Drawing for the job (mm, zero at the part's lowest x, y, z). A direction names the side the tool comes from. Round coordinates to 2 decimals unless told otherwise and drop trailing zeros. Write each loop counter-clockwise with the first axis right and the second up, starting at its lowest first coordinate (ties: lowest second). Pieces come first, ordered by that corner, then holes. Notation, with made-up numbers: M 45,75.25 L 53,75.25 A8 ccw 53,85.25 Z; hole C -26,83 d8. An arc over 180 degrees is marked long. Use a Markdown table: item, result. Add a question column.
1) Which spindle directions (+Z, -Z, +X, -X, +Y, -Y) get a long thin tool onto all of the face, cutting with end or side? Do the marked faces 1 and 2. Say none if no direction does.
2) Wall check: probe 1 along Y at (x, z) = (22.5, 4); probe 2 along X at (y, z) = (9, 77.5); probe 3 along Y at (x, z) = (7, 47). Give the ranges that are in metal, low to high.
3) Slice it at A-A on z = 74. Write the cut outline in (x, y), plus the area to 3 significant figures.
4) Slice it at B-B on y = 4. Write the cut outline in (x, z).
5) Drop flat-ended pins along their axis: P1, Ø14, axis at y = 8.5, z = 64.5, coming from the +X side; P2, Ø2, axis at y = 17.5, z = 56, coming from the +X side; P3, Ø5, axis at x = 34, z = 82, coming from the -Y side. Give the stop position or say it passes through.
6) Slice it at C-C on x = 42.5. Write the cut outline in (y, z).
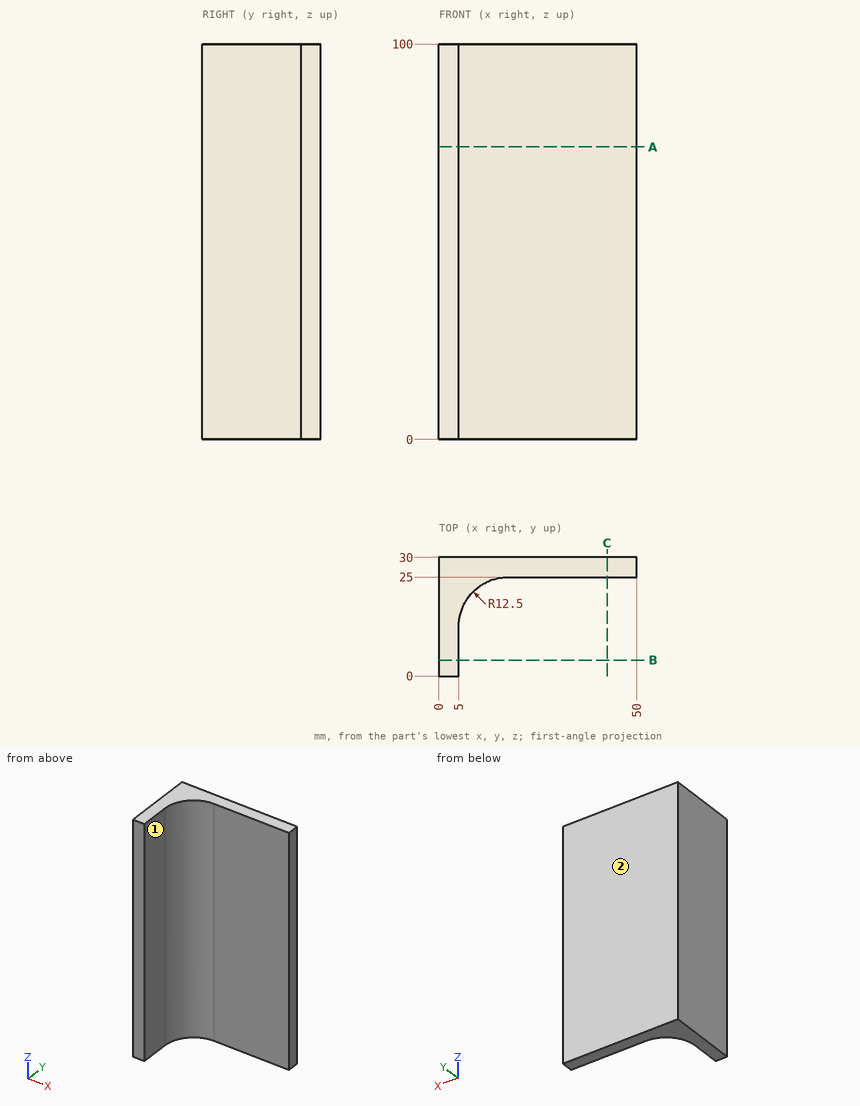
Entries:
| question | item | result |
|---|---|---|
| 1 | face 1 | +Z, -Z, +X, -Y |
| 1 | face 2 | +Z, -Z, +X, -X, +Y |
| 2 | probe 1 | y = 25 to 30 |
| 2 | probe 2 | x = 0 to 5 |
| 2 | probe 3 | y = 19.28 to 30 |
| 3 | outline | M 0,0 L 5,0 L 5,12.5 A12.5 cw 17.5,25 L 50,25 L 50,30 L 0,30 Z |
| 3 | area | 409 mm^2 |
| 4 | outline | M 0,0 L 5,0 L 5,100 L 0,100 Z |
| 5 | P1 | stops at x = 5.37 |
| 5 | P2 | stops at x = 6.53 |
| 5 | P3 | stops at y = 25 |
| 6 | outline | M 25,0 L 30,0 L 30,100 L 25,100 Z |
